Here's how the part is built. I have some questions about the finished solid (model axes, mm). Face numbers are marked on the shaded views. A direction names the side the tool comes from. Round coordinates to 2 decimals unless told otherwise and drop trailing zeros. Order: outer loops, then holes, each group sorted by start corner. A loop starts at its lowest first (then second) coordinate and runs counter-clockwise, first axis right, second up. Notation, with made-up numbers: (8.25, -23) - (57.25, -23) arc R22 ccw to (57.25, -11) - close; hole circle Ø7 at (46.25, 7). An arc over 180 degrees is marked (long way). Answer as a JSON object with one key per item and string values.
```python
from build123d import *

# Parameters (mm, degrees)
EXTRUDE_1_DEPTH     = 10
SKETCH_2_R          = 3
CUT_EXTRUDE_1_DEPTH = 2
SKETCH_3_R          = 3
CUT_EXTRUDE_2_DEPTH = 2


with BuildPart() as part:
    # 草图1 → 凸台-拉伸1 (new, symmetric)
    with BuildSketch(Plane.XY):
        Polygon((0, 0), (0, 20), (2, 20), (2, 2), (15, 2), (15, 0), align=None)
    extrude(amount=EXTRUDE_1_DEPTH, both=True)

    # 草图2 → 切除-拉伸1 (cut)
    with BuildSketch(Plane.ZY):
        with Locations((0, 10)):
            Circle(SKETCH_2_R)
    extrude(amount=-CUT_EXTRUDE_1_DEPTH, mode=Mode.SUBTRACT)

    # 草图3 → 切除-拉伸2 (cut)
    with BuildSketch(Plane.XZ):
        with Locations((5, 0)):
            Circle(SKETCH_3_R)
    extrude(amount=-CUT_EXTRUDE_2_DEPTH, mode=Mode.SUBTRACT)


solid = part.part
```
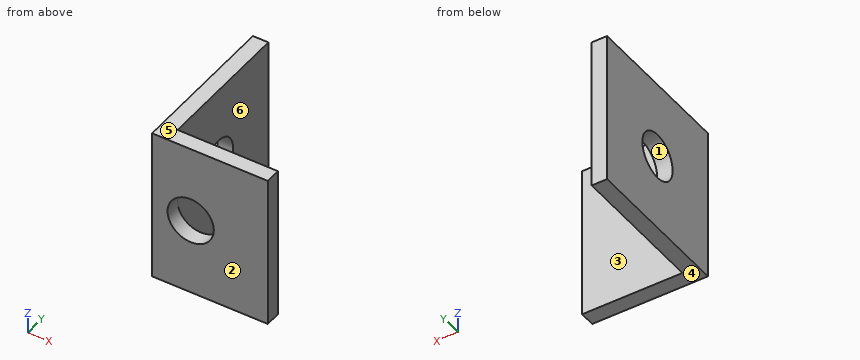
1. Imagine slicing it at A-A (y = 10). List the corners of the cut face in (x, z) for me.
Responses:
{"outline": "(0, -10) - (2, -10) - (2, -3) - (0, -3) - close; (0, 3) - (2, 3) - (2, 10) - (0, 10) - close"}
2. Thinking about a two-plate mould opening in Y: for the marked faces 1, 2, 3 and 4, which applies, pulls with the +Y half, pulls with the -Y half, needs draft (parallel to the pull), parting line crosses it, or undercut?
Responses:
{"face 1": "undercut", "face 2": "pulls with the -Y half", "face 3": "pulls with the +Y half", "face 4": "needs draft"}
3. Imagine slicing it at D-D (z = 5). List the corners of the cut face in (x, y) for me, plus the area to 3 significant figures.
Responses:
{"outline": "(0, 0) - (15, 0) - (15, 2) - (2, 2) - (2, 20) - (0, 20) - close", "area": "66.0 mm2"}
4. For the marked faces 5 and 6, which set-ups out of +Z, -Z, +X, -X, +Y, -Y let a thin tool reach every point of the face, with its end or its side?
Responses:
{"face 5": "+Z, +X, -X, +Y, -Y", "face 6": "+Z, -Z, +X, +Y"}
5. If I drill on L1, parallel to Y at x = 0.75, z = 0; L2, parallel to X at y = 1.2, z = 0; L3, parallel to Y at x = 8, z = 1.25, over which ranges is the centre line in solid material (lowest first)? Write a range as [from, to].
Responses:
{"L1": "[0, 7], [13, 20]", "L2": "[0, 2], [8, 15]", "L3": "[0, 2]"}
6. Imagine slicing it at C-C (z = -1.75). List the corners of the cut face in (x, y) for me, plus the area to 3 significant figures.
Responses:
{"outline": "(0, 0) - (2.56, 0) - (2.56, 2) - (2, 2) - (2, 7.56) - (0, 7.56) - close; (0, 12.44) - (2, 12.44) - (2, 20) - (0, 20) - close; (7.44, 0) - (15, 0) - (15, 2) - (7.44, 2) - close", "area": "46.5 mm2"}
7. For P1, Ø2, axis at x = 11, z = 0, coming from the -Y side; P2, Ø5, axis at y = 17.5, z = 5.5, coming from the +X side, each with a flat end and sliding along its axis, tell me the tip position at first contact or that it passes through.
Responses:
{"P1": "y = 0", "P2": "x = 2"}
